Design review of the part built by this model. Coordinates are the model's own, in mm. Face numbers are marked on the shaded views. A direction names the side the tool comes from. Coordinates: 2 decimals unless noted, no trailing zeros. Loops run counter-clockwise (first coordinate to the right, second up) from the corner with the lowest first, then second, coordinate; pieces in that order, holes last. Notation, with made-up numbers: (14.25, 66.5) - (62.25, 66.5) arc R20 cw to (62.25, 96.5) - close; hole circle Ø3 at (87.5, 30). An arc over 180 degrees is marked (long way). Return JSON: item names as keys, results as strings. Group by question number.
from build123d import *

# Parameters (mm, degrees)
AUFSATZ_LINEAR_AUSTRAGEN1_DEPTH = 303.9
SCHNITT_LINEAR_AUSTRAGEN1_DEPTH = 1.5
SCHNITT_LINEAR_AUSTRAGEN2_DEPTH = 1.5


with BuildPart() as part:
    # Skizze1 → Aufsatz-Linear austragen1 (new body)
    with BuildSketch(Plane(origin=(0, 0, 300), x_dir=(-1, 0, 0), z_dir=(0, 0, -1))):
        Polygon((461.5, -500), (500, -500), (500, -461.5), (501.5, -461.5), (501.5, -501.5), (461.5, -501.5), align=None)
    extrude(amount=AUFSATZ_LINEAR_AUSTRAGEN1_DEPTH)

    # Skizze2 → Schnitt-Linear austragen1 (cut)
    with BuildSketch(Plane.XZ.offset(501.5)):
        Polygon((-461.5, -3.9), (-501.5, -3.9), (-461.5, 36.1), align=None)
    extrude(amount=-SCHNITT_LINEAR_AUSTRAGEN1_DEPTH, mode=Mode.SUBTRACT)

    # Skizze3 → Schnitt-Linear austragen2 (cut)
    with BuildSketch(Plane.ZY.offset(501.5)):
        Polygon((-3.9, -461.5), (-3.9, -501.5), (36.1, -461.5), align=None)
    extrude(amount=-SCHNITT_LINEAR_AUSTRAGEN2_DEPTH, mode=Mode.SUBTRACT)


solid = part.part
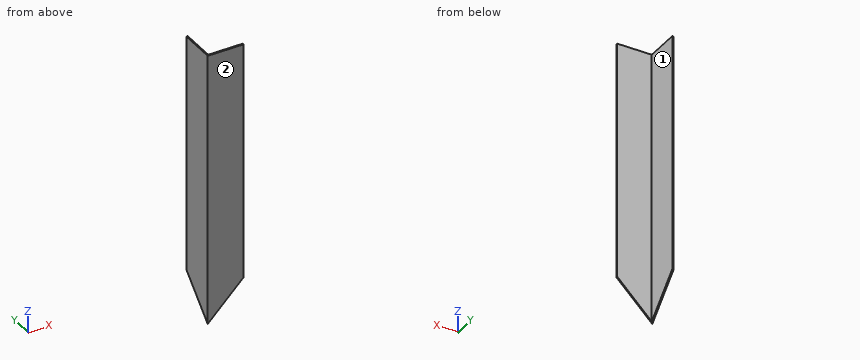
Item 1: For P1, Ø19, axis at y = -474, z = 77.5, coming from the +X side, flat-tipped, find the tip position at first contact; note if it passes through.
Item 2: For the marked faces 1 and 2, list the 3-axis set-ups (+Z, -Z, +X, -X, +Y, -Y) from which the entire face can be reached by the end or side of a thin tool; tool diameter is ignored.
Item 3: Add section D-D (z = 169.5). State the section outline as (x, y) points.
Item 4: To check wall thickness, follow line 1 (Y direction, x = -496.5, z = 45). State the ranges of the line that lie inside material, in increasing order. Write a range as from..to.
Item 5: Add section B-B (y = -484). State the section outline as (x, z) points.
Item 6: Add section C-C (x = -491). State the section outline as (y, z) points.
Item 7: Add section A-A (z = 15). State the section outline as (x, y) points.
Answers below:
{
 "1": {"P1": "stops at x = -500"},
 "2": {"face 1": "+Z, -Z, +X, +Y", "face 2": "+Z, -Z, +X, -X, -Y"},
 "3": {"outline": "(-501.5, -501.5) - (-461.5, -501.5) - (-461.5, -500) - (-500, -500) - (-500, -461.5) - (-501.5, -461.5) - close"},
 "4": {"line 1": "y = -501.5..-500"},
 "5": {"outline": "(-501.5, 13.6) - (-500, 13.6) - (-500, 300) - (-501.5, 300) - close"},
 "6": {"outline": "(-501.5, 6.6) - (-500, 6.6) - (-500, 300) - (-501.5, 300) - close"},
 "7": {"outline": "(-501.5, -501.5) - (-482.6, -501.5) - (-482.6, -500) - (-500, -500) - (-500, -482.6) - (-501.5, -482.6) - close"}
}
